Autodesk Inventor part; units mm, degrees
ref_plane "Work Plane1" through (104.775, 0, 0) normal (0, 0, -1) x (1, 0, 0)
ref_plane "YZ Plane" through (0, 0, 0) normal (1, 0, 0) x (0, 1, 0)
ref_plane "XZ Plane" through (0, 0, 0) normal (0, 1, 0) x (-1, 0, 0)
sketch "Skizze1" plane through (0, 0, 0) normal (0, 0, 1) x (1, 0, 0)
  line L0 (6.35, 0) -> (6.35, 1.4224)
  line L1 (6.35, 1.4224) -> (3.6957, 1.4224)
  line L2 (3.6957, 1.4224) -> (2.1082, 1.4224)
  line L3 (0, 2.7686) -> (0, 0.9092)
  line L4 (0, 0.9092) -> (1.397, 0.9092)
  line L5 (1.397, 0.9092) -> (1.9219, 0)
  line L6 (1.9219, 0) -> (6.35, 0)
  line L7 (0, 2.7686) -> (0.1596, 2.7686)
  line L8 (0.1596, 2.7686) -> (1.7082, 1.4224)
  line L9 (2.1082, 1.4224) -> (1.7082, 1.4224)
  line L10 (3.6957, 1.4224) -> (1.7082, 1.4224) construction
  line L11 (1.7082, 1.4224) -> (1.7082, 1.4224)
  line L12 (-1.27, 0) -> (7.62, 0)
  line L13 (0, -0.5537) -> (0, 3.3223)
  dimension "d0" = 6.35
  dimension "d1" = 2.6543
  dimension "d2" = 1.397
  dimension "d3" = 2.8448
  dimension "d6" = 1.7082
  dimension "d7" = 41
  dimension "d8" = 1.8184
  dimension "d9" = 60
  dimension "d10" = 5.5372
  dimension "d11" = 2.8448
  dimension "d12" = 1.5875
revolve "Körper" add sketch "Skizze1" angle 360 about axis through (1.9219, 0, 0) along (1, 0, 0) contours L6 L5 L4 L3 L7 L8 L9 L2 L1 L0
sketch "Skizze2" plane through (0, 0, 0) normal (-1, 0, 0) x (0, 0, 1)
  circle A0 centre (0, 0) radius 0.9092
  line L0 (0, -3.876) -> (0, 3.876)
  line L1 (-3.876, 0) -> (3.876, 0)
  line L2 (0.9092, 0) -> (0.4546, -0.7874)
  line L3 (0.4546, -0.7874) -> (-0.4546, -0.7874)
  line L4 (-0.4546, -0.7874) -> (-0.9092, 0)
  line L5 (-0.9092, 0) -> (-0.4546, 0.7874)
  line L6 (-0.4546, 0.7874) -> (0.4546, 0.7874)
  line L7 (0.4546, 0.7874) -> (0.9092, 0)
  point P0 (0, 0.9092)
extrude "Loch" add sketch "Skizze2" against normal up to next contours L7 A0 | A0 L2 | L6 L0 A0 | A0 L0 L3 | L0 L6 A0 | A0 L3 L0 | L4 A0 | A0 L5
thread "Gewinde"
chamfer "Fase1" distance 0.3785 distance2 0.7569 1 edges at (6.35, -1.4224, 0) measured on face at (6.35, -0.1427, 0.3949)
ref_plane "Work Plane1" through (104.775, 0, 0) normal (0, 0, -1) x (1, 0, 0)
equation "\"d15\" = GEL"
equation "\"d17\" = -0.5 * SPD + 0.5 * GD"
equation "\"d18\" = GUL"
equation "\"d0\" = NLG"
equation "\"d1\" = GEL"
equation "\"d2\" = INTI"
equation "\"d3\" = GD"
equation "\"d7\" = 0.5 * SEWI"
equation "\"d8\" = 1.1547 * SW"
equation "\"d10\" = KOD"
equation "\"d11\" = BDM"
equation "\"d12\" = GAL"
equation "\"NLG\" = 6.35"
equation "\"INTI\" = 1.397"
equation "\"GEL\" = 2.6543"
equation "\"GAL\" = 1.5875"
equation "\"KOH\" = 2.1082"
equation "\"KOD\" = 5.5372"
equation "\"GUL\" = 0.75692"
equation "\"SPD\" = 2.08788"
equation "\"BDM\" = NND"
equation "\"GD\" = NND"
equation "\"SEWI\" = 82deg"
equation "\"SW\" = 1.5748"
equation "\"TOA\" = 30deg"
equation "\"GD1\" = SPD"
equation "\"THREADDIA\" = 2.8448"
equation "\"HHPTC\" = 0.635"
equation "\"NND\" = 2.8448"
equation "\"E0\" = 1.155 * SW"
properties part number "ANSI B18.3 - 4-40 UNC x 0,25" material "Edelstahl"
Part model, mm, in its own coordinate system. A direction names the side the tool comes from. Coordinates: 2 decimals unless noted, no trailing zeros. Loops run counter-clockwise (first coordinate to the right, second up) from the corner with the lowest first, then second, coordinate; pieces in that order, holes last. Notation, with made-up numbers: M 79,38 L 134,38 A20 cw 134,65 Z; hole C -4.75,-31.75 d1. An arc over 180 degrees is marked long. Use a Markdown table: item, result. Add a question column.
Q1. Pin check, flat tips, straight feed: P1, Ø1.5, axis at y = 2, z = 1, coming from the +X side; P2, Ø1.5, axis at x = 1, z = -2, coming from the -Y side; P3, Ø0.5, axis at x = 0.5, z = 0, coming from the +Y side. Stop position of each tip, or through.
Q2. Cut at B-B (x = 3.25). Write the cut outline in (y, z).
Q3. Probe L1, parallel to Y at x = 0.75, z = -1.75; L2, parallel to X at y = -0.05, z = -1.95; L3, parallel to Y at x = 1.5, z = -0.5. List the from-to ranges inside material, lowest first.
Q4. Which spindle directions (+Z, -Z, +X, -X, +Y, -Y) get a long thin tool onto all of the face, cutting with end or side? Do faces 4 (the flat face through (0, -1, 1)), 5 (the flat face through (1, -0.787, 0)). Say none if no direction does.
Q5. Cut at A-A (x = 1). Write the cut outline in (y, z), and give its area (3 significant figures).
Q6. Mould opens along Z. For faces 1 (the flat face through (1, 0.787, 0)), 2 (the cylindrical face through (3.62, -0.31, 1.39)), 3 (the flat face through (6.35, 0, 0)) say: +Z half, -Z half, draft (parallel to the pull), parting line (faces both ways), or undercut.
Worked out:
| question | item | result |
|---|---|---|
| 1 | P1 | stops at x = 1.63 |
| 1 | P2 | stops at y = -2.04 |
| 1 | P3 | stops at y = 2.69 |
| 2 | outline | C 0,0 d2.84 |
| 3 | L1 | y = -1.42 to 1.42 |
| 3 | L2 | x = 0 to 1.1 |
| 3 | L3 | y = -1.52 to -0.53, 0.53 to 1.52 |
| 4 | face 4 | +Z, -Z, -X, +Y, -Y |
| 4 | face 5 | -X |
| 5 | outline | C 0,0 d4.08; hole M -0.79,-0.45 L 0,-0.91 L 0.79,-0.45 L 0.79,0.45 L 0,0.91 L -0.79,0.45 Z |
| 5 | area | 10.9 mm2 |
| 6 | face 1 | undercut |
| 6 | face 2 | parting line |
| 6 | face 3 | draft |
